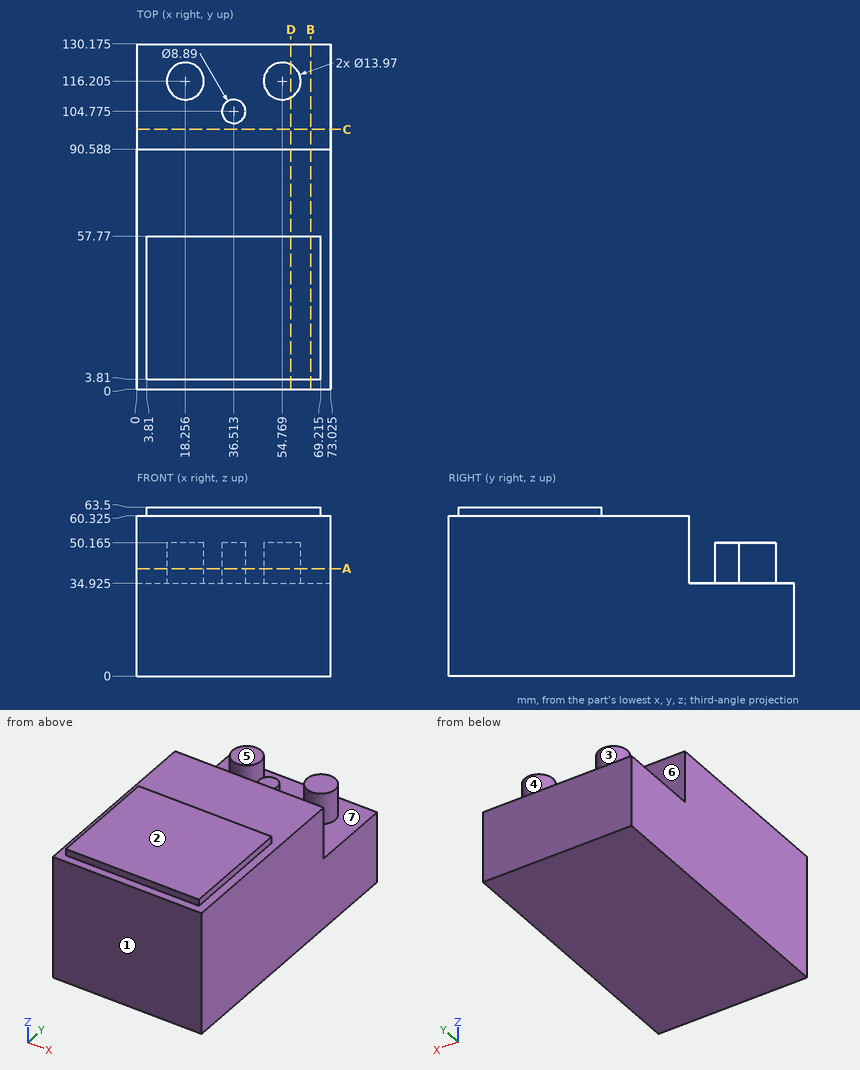
Geometry: see drawing. Coordinates: mm, zero at the bounding-box minimum. A direction names the side the tool comes from. Coordinates: 2 decimals unless noted, no trailing zeros. Write each loop counter-clockwise with the first axis right and the second up, starting at its lowest first coordinate (ties: lowest second). Pieces come first, ordered by that corner, then holes. Notation, with made-up numbers: M 8,-17.75 L 54,-17.75 A27 ccw 54,12.25 Z; hole C 80,23.25 d7. An arc over 180 degrees is marked long. Answer as a JSON object with one key per item and string values.
1. Cut plane A-A on z = 40.5. Output: boundary loops of the cut face in (x, y) (1 decimal), plus the area to 3 significant figures.
Evaluation:
{"outline": "M 0,0 L 73,0 L 73,90.6 L 0,90.6 Z; C 18.3,116.2 d14; C 36.5,104.8 d8.9; C 54.8,116.2 d14", "area": "6,980 mm^2"}
2. Cut plane B-B on x = 65.5. Output: boundary loops of the cut face in (y, z) (1 decimal), plus the area to 3 significant figures.
Evaluation:
{"outline": "M 0,0 L 130.2,0 L 130.2,34.9 L 90.6,34.9 L 90.6,60.3 L 57.8,60.3 L 57.8,63.5 L 3.8,63.5 L 3.8,60.3 L 0,60.3 Z", "area": "7,020 mm^2"}
3. Contact query for flat-ended pins moving along their axis: P1, Ø10, axis at x = 36, y = 106.5, coming from the +Z side (1 decimal); P2, Ø8, axis at x = 61, y = 59.5, coming from the +Z side; P3, Ø3.5, axis at x = 39, z = 62.5, coming from the +Y side; P4, Ø12.5, axis at x = 19.5, z = 53.5, coming from the +Y side. Output: stop coordinate, or through.
Evaluation:
{"P1": "z = 50.2", "P2": "z = 63.5", "P3": "y = 57.77", "P4": "y = 123.19"}
4. Cut plane C-C on y = 98. Output: boundary loops of the cut face in (x, z) (1 decimal).
Evaluation:
{"outline": "M 0,0 L 73,0 L 73,34.9 L 0,34.9 Z"}
5. Access query for the marked faces 5, 6 and 7. Directions: +Z, -Z, +X, -X, +Y, -Y. A direction counts if a zero-diameter tool reaches every point of the face in a straight line with its end or side. Return the directions, or none.
Evaluation:
{"face 5": "+Z, +X, -X, +Y", "face 6": "+Z, +X, -X", "face 7": "+Z"}
6. Cut plane D-D on x = 58. Output: boundary loops of the cut face in (y, z) (1 decimal).
Evaluation:
{"outline": "M 0,0 L 130.2,0 L 130.2,34.9 L 122.4,34.9 L 122.4,50.2 L 110,50.2 L 110,34.9 L 90.6,34.9 L 90.6,60.3 L 57.8,60.3 L 57.8,63.5 L 3.8,63.5 L 3.8,60.3 L 0,60.3 Z"}
7. Ray query, L1, parallel to Y at x = 3.5, z = 58; L2, parallel to Y at x = 51, z = 40.5 (1 decimal); L3, parallel to Y at x = 35, z = 43.5 (1 decimal). Return the intervals inside material, ascending.
Evaluation:
{"L1": "0 to 90.59", "L2": "0 to 90.6, 110.3 to 122.1", "L3": "0 to 90.6, 100.6 to 109"}
8. Draft query along Y for the marked faces 1, 2, 3 and 4. Return one class per face: released by +Y, released by -Y, zero draft, split by the parting line, or undercut.
Evaluation:
{"face 1": "released by -Y", "face 2": "zero draft", "face 3": "undercut", "face 4": "undercut"}
